from build123d import *

# Parameters (mm, degrees)
SKETCH1_R           = 10
SKETCH1_R_2         = 7
BOSS_EXTRUDE1_DEPTH = 100.5
SKETCH2_R           = 8
CUT_EXTRUDE1_DEPTH  = 10
SKETCH3_R           = 8
CUT_EXTRUDE2_DEPTH  = 10
SKETCH4_W           = 1.3
SKETCH4_H           = 0.5
SKETCH5_R           = 1.5
CUT_EXTRUDE3_DEPTH  = 10
CHAMFER1_SIZE       = 0.5
FILLET1_R           = 0.3


with BuildPart() as part:
    # Sketch1 → Boss-Extrude1 (new body)
    with BuildSketch(Plane(origin=(0, 0, 0), x_dir=(0, 0, -1), z_dir=(1, 0, 0))):
        Circle(SKETCH1_R)
        Circle(SKETCH1_R_2, mode=Mode.SUBTRACT)
    extrude(amount=BOSS_EXTRUDE1_DEPTH)

    # Sketch2 → Cut-Extrude1 (cut)
    with BuildSketch(Plane.ZY):
        Circle(SKETCH2_R)
    extrude(amount=-CUT_EXTRUDE1_DEPTH, mode=Mode.SUBTRACT)

    # Sketch3 → Cut-Extrude2 (cut)
    with BuildSketch(Plane(origin=(100.5, 0, 0), x_dir=(0, 0, -1), z_dir=(1, 0, 0))):
        Circle(SKETCH3_R)
    extrude(amount=-CUT_EXTRUDE2_DEPTH, mode=Mode.SUBTRACT)

    # Sketch4 → Cut-Revolve1 (revolve, cut)
    with BuildSketch(Plane.XY):
        with Locations((69.65, 9.75)):
            Rectangle(SKETCH4_W, SKETCH4_H)
    revolve(axis=Axis((100.5, 0, 0), (-1, 0, 0)), mode=Mode.SUBTRACT)

    # Sketch5 → Cut-Extrude3 (cut, symmetric)
    with BuildSketch(Plane(origin=(0, 0, 0), x_dir=(1, 0, 0), z_dir=(0, 1, 0))):
        with Locations((24.5, 0)):
            Circle(SKETCH5_R)
    extrude(amount=CUT_EXTRUDE3_DEPTH, both=True, mode=Mode.SUBTRACT)

    # Chamfer1
    chamfer1_edges = [part.edges().sort_by_distance(p)[0] for p in [
        (0, 0, 10),
        (100.5, 0, 10),
    ]]
    chamfer(chamfer1_edges, length=CHAMFER1_SIZE)

    # Fillet1
    fillet1_edges = [part.edges().sort_by_distance(p)[0] for p in [
        (10, 0, -8),
        (90.5, 0, 8),
    ]]
    fillet(fillet1_edges, radius=FILLET1_R)


solid = part.part
Work out the finished part from the listing and answer in its coordinate system (mm). A direction names the side the tool comes from. Round coordinates to 2 decimals unless told otherwise and drop trailing zeros. Write each loop counter-clockwise with the first axis right and the second up, starting at its lowest first coordinate (ties: lowest second). Pieces come first, ordered by that corner, then holes.
1) Given pin 1 Ø1 at (x, y) = (53.5, -2.5) entering from -Z; pin 2 Ø2.5 at (x, z) = (24.5, 0) entering from -Y; pin 3 Ø5 at (x, z) = (26, -5) entering from +Y; pin 4 Ø4 at (x, y) = (78.5, -4.5) entering from +Z, each flat-ended and moving along its own axis, determine where each tip first touches the part or whether it passes through.
2) The mould has two halves that part along X. Classify faces 1 (the flat face through (100.5, -7, 4.3)), 2 (the cylindrical face through (95.72, -7.81, 1.73)), 3 (the cylindrical face through (23, 8, 0)): pulls with the +X half, pulls with the -X half, needs draft (parallel to the pull), parting line crosses it, or undercut.
3) A tool of negligible diameter and unlimited length cuts with its end or side. For faces 4 (the flat face through (10, -7, 2)), 5 (the flat face through (70.3, -9, 4)), 6 (the flat face through (90.5, -7, -2)), from which of +Z, -Z, +X, -X, +Y, -Y can it reach the whole face along a straight path? Write none if from no direction.
4) A cutting plane is placed at C-C (x = 94). Give the vertices of the cut face in (y, z), plus the area to 3 significant figures.
5) A cutting plane is placed at B-B (x = 24.5). Give the vertices of the cut face in (y, z), plus the area to 3 significant figures.
6) Straight lines are drawn through the part: line 1 (Y direction, x = 56.5, z = 0); line 2 (Z direction, x = 24.5, y = -7.6); line 3 (Z direction, x = 24.5, y = 8.3). For each, find the intervals that lie inside material, in ascending order.
Completed:
1. pin 1: stops at z = -9.8
1. pin 2: passes through
1. pin 3: stops at y = 9.68
1. pin 4: stops at z = 9.68
2. face 1: pulls with the +X half
2. face 2: needs draft
2. face 3: undercut
3. face 4: -X
3. face 5: none
3. face 6: +X
4. outline: circle Ø20 at (0, 0); hole circle Ø16 at (0, 0)
4. area: 113 mm2
5. outline: (-9.89, -1.5) arc R10 ccw to (9.89, -1.5) - (6.84, -1.5) arc R7 cw to (-6.84, -1.5) - close; (-9.89, 1.5) - (-6.84, 1.5) arc R7 cw to (6.84, 1.5) - (9.89, 1.5) arc R10 ccw to start
5. area: 142 mm2
6. line 1: y = -10 to -7, 7 to 10
6. line 2: z = -6.5 to -1.5, 1.5 to 6.5
6. line 3: z = -5.58 to -1.5, 1.5 to 5.58
